Could you check a few things on this model? Use its own coordinates, in mm. A direction names the side the tool comes from. Give positions to 0.01 mm unless a question says otherwise; leave off trailing zeros. Loops run counter-clockwise (first coordinate to the right, second up) from the corner with the lowest first, then second, coordinate; pieces in that order, holes last. Notation, with made-up numbers: M -32,-16 L 20,-16 A14 cw 20,8 Z; hole C 22.25,-20.5 d6. An arc over 180 degrees is marked long. Return JSON: item names as keys, results as strings. Group by question number.
1. If we mould it in two halves opening along X, with no side actions, what happens to faces 5 (the flat face through (-16, 5.4, 4)), 6 (the flat face through (0, 6, 0)), 7 (the flat face through (-19.25, 4, 4))? For each: +X half, -X half, draft (parallel to the pull), parting line (faces both ways), or undercut.
2. Please list where these lines run through material, in increasing order: line 1 (X direction, y = 2, z = 2.25); line 2 (Y direction, x = 19, z = 3.25); line 3 (X direction, y = 3.5, z = 0.5).
3. If we section it at A-A (y = -1): Write out the boundary of the cut face in (x, z).
4. If we section it at D-D (z = 5.5): State how many separate pieces and enclosed holes the cut face has, plus the area to 3 significant figures.
5. For pin 1 (1.7 mm diameter, centred on x = -17, z = 3.5, fed in from -Y); pin 2 (1 mm diameter, centred on x = 3, z = 2, fed in from +Y); pin 3 (4 mm diameter, centred on x = 0, z = 1.5, fed in from -Y), each with a flat end and sliding along its axis, tell me the tip position at first contact or that it passes through.
6. For faces 1 (the flat face through (19.25, 4, 4)), 2 (the flat face through (14.25, 8, 4)), 3 (the flat face through (21, -3, 4)), 4 (the flat face through (5.5, 1, 4)), which set-ups out of +Z, -Z, +X, -X, +Y, -Y let a thin tool reach every point of the face, with its end or its side?
7. If we section it at B-B (x = 15): Write out the boundary of the cut face in (y, z).
8. If we section it at C-C (y = 2): Write out the boundary of the cut face in (x, z).
```python
from build123d import *

# Parameters (mm, degrees)
SKETCH_W  = 5.6
SKETCH_H  = 2.4
PAD_DEPTH = 8


with BuildPart() as part:
    # Sketch → Pad (new body)
    with BuildSketch(Plane.XY):
        with BuildLine():
            Line((-22.25, -3), (-19.25, -3))
            Line((-19.25, -3), (-19.25, 0))
            Line((-19.25, 0), (-10.5, 0))
            Line((-10.5, 0), (-10.5, 2.5))
            ThreePointArc((-5.5, 2.5), (-8, 5), (-10.5, 2.5))
            Line((-5.5, 2.5), (-5.5, 0))
            Line((-5.5, 0), (-2.5, 0))
            Line((-2.5, 0), (-2.5, 2.5))
            ThreePointArc((2.5, 2.5), (0, 5), (-2.5, 2.5))
            Line((2.5, 2.5), (2.5, 0))
            Line((2.5, 0), (5.5, 0))
            Line((5.5, 0), (5.5, 2.5))
            ThreePointArc((10.5, 2.5), (8, 5), (5.5, 2.5))
            Line((10.5, 2.5), (10.5, 0))
            Line((10.5, 0), (19.25, 0))
            Line((19.25, 0), (19.25, -3))
            Line((19.25, -3), (22.25, -3))
            Line((22.25, -3), (22.25, 9))
            Line((22.25, 9), (14.25, 9))
            Line((14.25, 9), (14.25, 7))
            Line((14.25, 7), (-19.25, 7))
            Line((-19.25, 7), (-19.25, 10))
            Line((-19.25, 10), (-22.25, 10))
            Line((-22.25, 10), (-22.25, -3))
        make_face()
        with Locations((-16.45, 4.2)):
            Rectangle(SKETCH_W, SKETCH_H, mode=Mode.SUBTRACT)
        with Locations((16.45, 4.2)):
            Rectangle(SKETCH_W, SKETCH_H, mode=Mode.SUBTRACT)
    extrude(amount=PAD_DEPTH)


solid = part.part
```
Answer:
{
 "1": {"face 5": "undercut", "face 6": "draft", "face 7": "undercut"},
 "2": {"line 1": "x = -22.25 to -10.5, -5.5 to -2.5, 2.5 to 5.5, 10.5 to 22.25", "line 2": "y = 0 to 3, 5.4 to 9", "line 3": "x = -22.25 to -19.25, -13.65 to -10.29, -5.71 to -2.29, 2.29 to 5.71, 10.29 to 13.65, 19.25 to 22.25"},
 "3": {"outline": "M -22.25,0 L -19.25,0 L -19.25,8 L -22.25,8 Z; M 19.25,0 L 22.25,0 L 22.25,8 L 19.25,8 Z"},
 "4": {"separate pieces": "1", "enclosed holes": "2", "area": "261 mm²"},
 "5": {"pin 1": "stops at y = 0", "pin 2": "stops at y = 7", "pin 3": "stops at y = 4"},
 "6": {"face 1": "+Z, -Z", "face 2": "+Z, -Z, +Y", "face 3": "+Z, -Z, +X, -X, -Y", "face 4": "+Z, -Z, -Y"},
 "7": {"outline": "M 0,0 L 3,0 L 3,8 L 0,8 Z; M 5.4,0 L 9,0 L 9,8 L 5.4,8 Z"},
 "8": {"outline": "M -22.25,0 L -10.5,0 L -10.5,8 L -22.25,8 Z; M -5.5,0 L -2.5,0 L -2.5,8 L -5.5,8 Z; M 2.5,0 L 5.5,0 L 5.5,8 L 2.5,8 Z; M 10.5,0 L 22.25,0 L 22.25,8 L 10.5,8 Z"}
}
